Verification items for this drawing (mm, ordinates from the low corner). Round coordinates to 2 decimals unless told otherwise and drop trailing zeros. Order: outer loops, then holes, each group sorted by start corner. A loop starts at its lowest first (then second) coordinate and runs counter-clockwise, first axis right, second up. Notation, with made-up numbers: (-33, -3) - (-10, -3) arc R32 ccw to (-10, 29) - close; hole circle Ø8 at (-40, 52.5). An arc over 180 degrees is marked (long way). One line per question, with ' | ' between items. Start each with the question number.
Q1. Sectioned sample at B-B, the plane x = 50. Enter the section's corners in (y, z), then the cut area to 3 significant figures.
Q2. Sectioned sample at C-C, the plane y = 6.5. Enter the section's corners in (x, z).
Q3. Gauge pin test, flat ends, axial feed: P1, Ø3, axis at x = 63.5, y = 2.5, coming from the -Z side; P2, Ø2, axis at y = 9, z = 44.5, coming from the +X side. Record the tip position at first contact, or that the pin passes through.
Q4. Material ranges on line 1 along X through (y, z) = (3, 50); line 2 along Z through (x, y) = (38, 5.25), recorded low to high.
Q5. Mould release check, pull along Z, two halves, no side actions. Record for the marked faces 1, 2 and 3: +Z half, -Z half, draft (parallel to the pull), parting line (faces both ways), or undercut.
Q6. Sectioned sample at A-A, the plane z = 50. Enter the section's corners in (x, y).
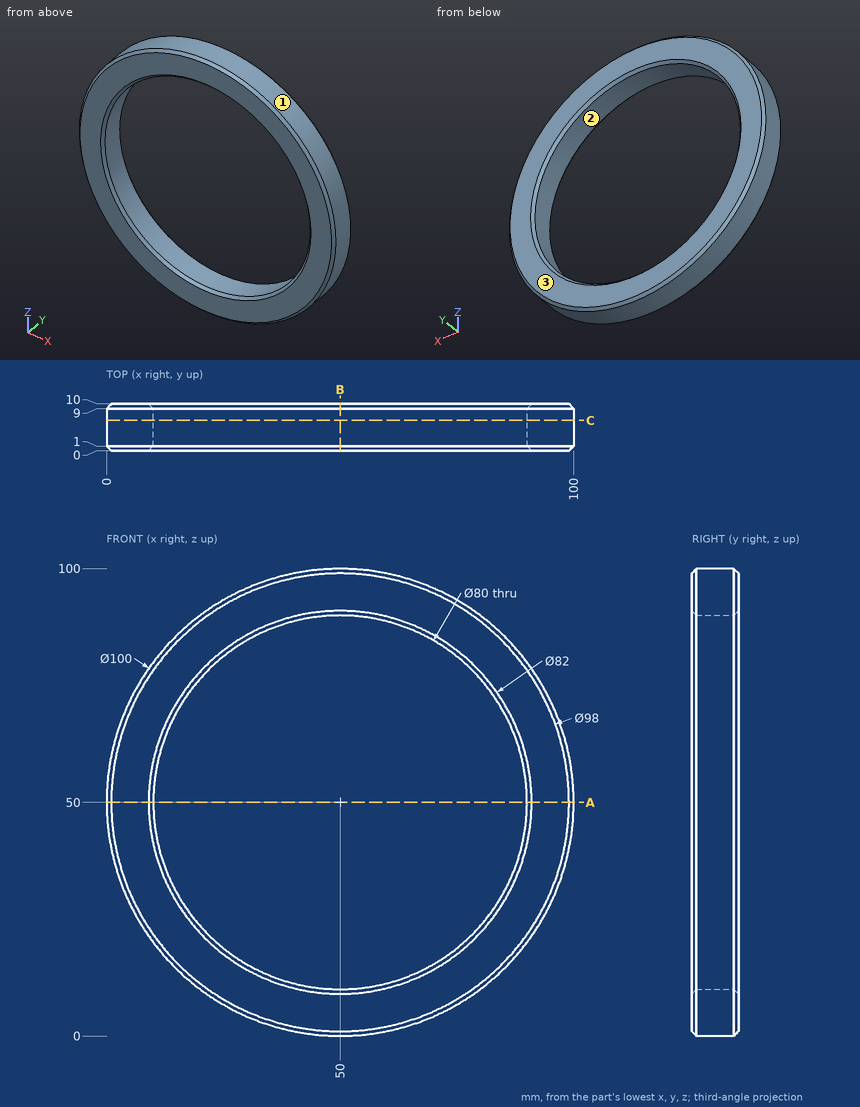
Determined:
1) outline: (0, 1) - (1, 0) - (9, 0) - (10, 1) - (10, 9) - (9, 10) - (1, 10) - (0, 9) - close; (0, 91) - (1, 90) - (9, 90) - (10, 91) - (10, 99) - (9, 100) - (1, 100) - (0, 99) - close | area: 196 mm2
2) outline: circle Ø100 at (50, 50); hole circle Ø80 at (50, 50)
3) P1: stops at z = 1.46 | P2: stops at x = 99.8
4) line 1: x = 0 to 10, 90 to 100 | line 2: z = 1.46 to 11.84, 88.16 to 98.54
5) face 1: parting line | face 2: undercut | face 3: draft
6) outline: (0, 1) - (1, 0) - (9, 0) - (10, 1) - (10, 9) - (9, 10) - (1, 10) - (0, 9) - close; (90, 1) - (91, 0) - (99, 0) - (100, 1) - (100, 9) - (99, 10) - (91, 10) - (90, 9) - close
